Design review of the part built by this model. Coordinates are the model's own, in mm. Face numbers are marked on the shaded views. A direction names the side the tool comes from. Coordinates: 2 decimals unless noted, no trailing zeros. Write each loop counter-clockwise with the first axis right and the second up, starting at its lowest first coordinate (ties: lowest second). Pieces come first, ordered by that corner, then holes. Notation, with made-up numbers: (36.5, 27.5) - (66.5, 27.5) arc R20 ccw to (66.5, 52.5) - close; hole circle Ø2 at (33.5, 13.25). An arc over 180 degrees is marked (long way). Use a Markdown table: item, result.
from build123d import *

# Parameters (mm, degrees)
CROQUIS1_W              = 30
CROQUIS1_H              = 35
CROQUIS1_R              = 2
SALIENTE_EXTRUIR1_DEPTH = 10
CROQUIS2_W              = 10
CROQUIS2_H              = 4
CORTAR_EXTRUIR1_DEPTH   = 41
REDONDEO1_R             = 5
CROQUIS3_R              = 1.5
CORTAR_EXTRUIR2_DEPTH   = 10
CROQUIS4_W              = 6
CROQUIS4_H              = 2
SALIENTE_EXTRUIR2_DEPTH = 3
CROQUIS5_W              = 1.5
CROQUIS5_H              = 1.5
CORTAR_EXTRUIR3_DEPTH   = 3


with BuildPart() as part:
    # Croquis1 → Saliente-Extruir1 (new body)
    with BuildSketch(Plane(origin=(0, 0, 0), x_dir=(1, 0, 0), z_dir=(0, 1, 0))):
        with Locations((15, 17.5)):
            Rectangle(CROQUIS1_W, CROQUIS1_H)
        with Locations(Location((7.5, 5, 0), (0, 0, 270))):
            Circle(CROQUIS1_R, mode=Mode.SUBTRACT)
        with Locations(Location((22.5, 5, 0), (0, 0, 270))):
            Circle(CROQUIS1_R, mode=Mode.SUBTRACT)
    extrude(amount=SALIENTE_EXTRUIR1_DEPTH)

    # Croquis2 → Cortar-Extruir1 (cut)
    with BuildSketch(Plane(origin=(30, 0, 0), x_dir=(0, 0, -1), z_dir=(1, 0, 0))):
        with Locations((30, 5)):
            Rectangle(CROQUIS2_W, CROQUIS2_H)
    extrude(amount=-CORTAR_EXTRUIR1_DEPTH, mode=Mode.SUBTRACT)

    # Redondeo1
    redondeo1_edges = [part.edges().sort_by_distance(p)[0] for p in [
        (30, 5, 0),
        (0, 5, 0),
    ]]
    fillet(redondeo1_edges, radius=REDONDEO1_R)

    # Croquis3 → Cortar-Extruir2 (cut)
    with BuildSketch(Plane(origin=(0, 10, 0), x_dir=(1, 0, 0), z_dir=(0, 1, 0))):
        with Locations(Location((15, 15, 0), (0, 0, 270))):
            Circle(CROQUIS3_R)
    extrude(amount=-CORTAR_EXTRUIR2_DEPTH, mode=Mode.SUBTRACT)

    # Croquis4 → Saliente-Extruir2 (add)
    with BuildSketch(Plane(origin=(0, 10, 0), x_dir=(1, 0, 0), z_dir=(0, 1, 0))):
        with Locations((15, 17.5)):
            Rectangle(CROQUIS4_W, CROQUIS4_H)
    extrude(amount=SALIENTE_EXTRUIR2_DEPTH)

    # Croquis5 → Cortar-Extruir3 (cut)
    with BuildSketch(Plane.XY.offset(-16.5)):
        with Locations((17.25, 10.75)):
            Rectangle(CROQUIS5_W, CROQUIS5_H)
        with Locations((12.75, 10.75)):
            Rectangle(CROQUIS5_W, CROQUIS5_H)
    extrude(amount=-CORTAR_EXTRUIR3_DEPTH, mode=Mode.SUBTRACT)


solid = part.part
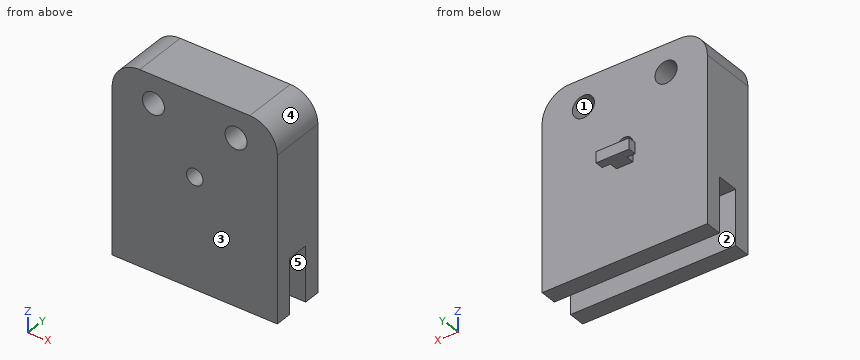
(1) Draft analysis for pull direction Y (two halves, no side actions). For the marked faces 1, 2 and 3, state which applies: +Y half, -Y half, draft (parallel to the pull), parting line (faces both ways), or undercut.
Determined:
| item | result |
|---|---|
| face 1 | draft |
| face 2 | undercut |
| face 3 | -Y half |
(2) Take a section at B-B on x = 22.5. Write out the cut boundary in (y, z).
Determined:
| item | result |
|---|---|
| outline | (0, -35) - (3, -35) - (3, -25) - (7, -25) - (7, -35) - (10, -35) - (10, -7) - (0, -7) - close; (0, -3) - (10, -3) - (10, 0) - (0, 0) - close |
(3) For pin 1 (4 mm diameter, centred on x = 13, z = -4, fed in from -Y); pin 2 (1.2 mm diameter, centred on y = 11, z = -17, fed in from -X); pin 3 (11 mm diameter, centred on x = 19.5, z = -30, fed in from +Y); pin 4 (1.5 mm diameter, centred on x = 16, y = 12, fed in from -Z), all flat-tipped, find the tip position at first contact; note any pin that passes through.
Determined:
| item | result |
|---|---|
| pin 1 | y = 0 |
| pin 2 | x = 12 |
| pin 3 | y = 10 |
| pin 4 | z = -18.5 |
(4) For L1, parallel to Z at x = 15, y = 8; L2, parallel to Y at x = 7.25, z = -27.5; L3, parallel to X at y = 3.75, z = -15, list the stretches that pass through material, from the lowest coordinate up. Write a range as from..to.
Determined:
| item | result |
|---|---|
| L1 | -35..-16.5, -13.5..0 |
| L2 | 0..3, 7..10 |
| L3 | 0..13.5, 16.5..30 |
(5) Take a section at C-C on y = 1.5. Write out the cut boundary in (x, z), and give its area (3 significant figures).
Determined:
| item | result |
|---|---|
| outline | (0, -35) - (30, -35) - (30, -5) arc R5 ccw to (25, 0) - (5, 0) arc R5 ccw to (0, -5) - close; hole circle Ø4 at (7.5, -5); hole circle Ø3 at (15, -15); hole circle Ø4 at (22.5, -5) |
| area | 1,010 mm2 |
(6) Machinability: for the marked faces 4 and 5, which of the approach directions +Z, -Z, +X, -X, +Y, -Y give a long, thin tool a straight path to every point of the face, cutting with its end or side? Answer none if there is none.
Determined:
| item | result |
|---|---|
| face 4 | +Z, +X, +Y, -Y |
| face 5 | -Z, +X, -X |
(7) Take a section at D-D on z = -29.5. Write out the cut boundary in (x, y).
Determined:
| item | result |
|---|---|
| outline | (0, 0) - (30, 0) - (30, 3) - (0, 3) - close; (0, 7) - (30, 7) - (30, 10) - (0, 10) - close |
(8) Take a section at A-A on z = -15. Write out the cut boundary in (x, y).
Determined:
| item | result |
|---|---|
| outline | (0, 0) - (13.5, 0) - (13.5, 10) - (0, 10) - close; (16.5, 0) - (30, 0) - (30, 10) - (16.5, 10) - close |
